Part print with two shaded views. Sizes in mm from the minimum x, y, z corner. A direction names the side the tool comes from. Give positions to 0.01 mm unless a question says otherwise; leave off trailing zeros. Write each loop counter-clockwise with the first axis right and the second up, starting at its lowest first coordinate (ties: lowest second). Pieces come first, ordered by that corner, then holes.
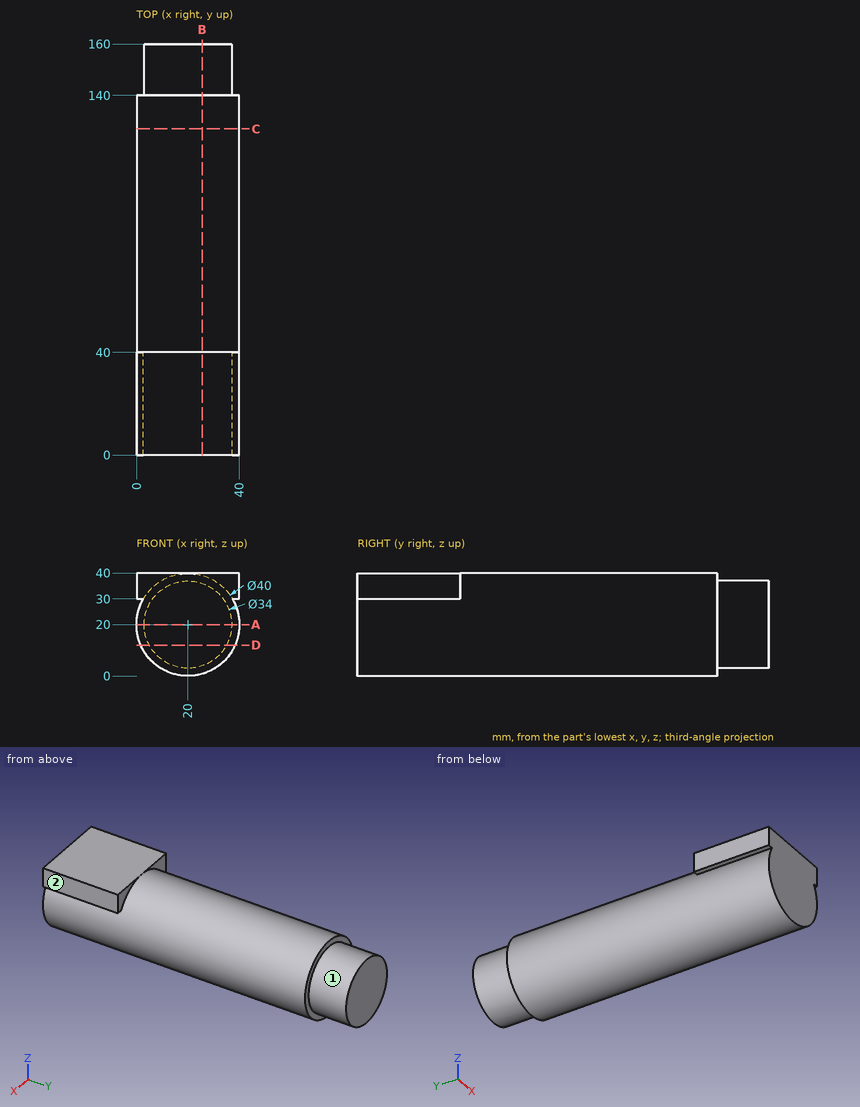
1) Saw through at D-D (z = 12). Write the cut outline in (x, y).
Check result:
outline: (1.67, 0) - (38.33, 0) - (38.33, 140) - (35, 140) - (35, 160) - (5, 160) - (5, 140) - (1.67, 140) - close
2) Saw through at C-C (y = 127). Write the cut outline in (x, z), and give its area (3 significant figures).
Check result:
outline: circle Ø40 at (20, 20)
area: 1,260 mm2
3) 3-axis set-ups, long thin cutter, end or side, ignore diameter. For the marked faces 1 and 2: which of +Z, -Z, +X, -X, +Y, -Y reach the whole face in a straight line?
Check result:
face 1: +Y
face 2: +Z, -Z, +X, +Y, -Y
4) Saw through at A-A (z = 20). Write the cut outline in (x, y), and give its area (3 significant figures).
Check result:
outline: (0, 0) - (40, 0) - (40, 140) - (37, 140) - (37, 160) - (3, 160) - (3, 140) - (0, 140) - close
area: 6,280 mm2
5) Drill centre lines: L1, parallel to Y at x = 37, z = 36; L2, parallel to Y at x = 6, z = 9; L3, parallel to X at y = 106, z = 30.5. Where is each one in solid material? Low to high.
Check result:
L1: y = 0 to 40
L2: y = 0 to 140
L3: x = 2.98 to 37.02
6) Saw through at B-B (x = 25.5). Write the cut outline in (y, z).
Check result:
outline: (0, 0.77) - (140, 0.77) - (140, 3.91) - (160, 3.91) - (160, 36.09) - (140, 36.09) - (140, 39.23) - (40, 39.23) - (40, 40) - (0, 40) - close
7) Flat gauge pins, fed straight in: P1, Ø3, axis at y = 50.5, z = 16, coming from the +X side; P2, Ø8, axis at y = 119.5, z = 14, coming from the -X side; P3, Ø3, axis at x = 34, z = 34, coming from the +Y side; P4, Ø10, axis at x = 24.5, y = 45, coming from the -Z side. Where does each tip first touch, or does it go through?
Check result:
P1: stops at x = 39.84
P2: stops at x = 0.1
P3: stops at y = 140
P4: stops at z = 0
